```python
from build123d import *

# Parameters (mm, degrees)
F0_W     = 38.1
F0_H     = 25.4
F0_R     = 2.286
F1_DEPTH = 304.8
F2_R     = 12.7
F3_DEPTH = 25.401


with BuildPart() as f1:
    # F0 (on Front) → F1 (new body)
    with BuildSketch(Plane.XZ):
        with Locations((19.05, 12.7)):
            Rectangle(F0_W, F0_H)
        with Locations((9.906, 12.7)):
            Circle(F0_R, mode=Mode.SUBTRACT)
        with Locations((28.194, 12.7)):
            Circle(F0_R, mode=Mode.SUBTRACT)
    extrude(amount=F1_DEPTH)

    # F2 (on Top) → F3 (cut, through all)
    with BuildSketch(Plane.XY):
        with Locations((17.78, -241.3)):
            Circle(F2_R)
        with Locations((17.78, -63.5)):
            Circle(F2_R)
    extrude(amount=F3_DEPTH, mode=Mode.SUBTRACT)


solid = f1.part
```
Model file for the job. Use its own axes, mm. Coordinates: 2 decimals unless noted, no trailing zeros. Loops run counter-clockwise (first coordinate to the right, second up) from the corner with the lowest first, then second, coordinate; pieces in that order, holes last. Notation, with made-up numbers: (24, 4) - (77, 4) arc R31 cw to (77, 31) - close; hole circle Ø3 at (-14.75, 83). An arc over 180 degrees is marked (long way). Write item = value, one per line. Start each with the question number.
Item 1: Saw through at A-A, the plane x = 17.78. List the corners of the cut face in (y, z), then the cut area to 3 significant figures.
Item 2: Drop a flat-ended pin along its axis: pin 1 Ø5.5 at (x, z) = (28.194, 12.7) entering from -Y. Give the stop position or say it passes through.
Item 3: Saw through at B-B, the plane y = -150. List the corners of the cut face in (x, z), then the cut area to 3 significant figures.
Item 4: Wall check: probe 1 along Y at (x, z) = (18, 19.5); probe 2 along X at (y, z) = (-257, 13); probe 3 along X at (y, z) = (-216.5, 12.25). Give the ranges that are in metal, low to high. Write a range as [from, to].
Item 5: Saw through at C-C, the plane z = 22.75. List the corners of the cut face in (x, y), then the cut area to 3 significant figures.
Item 6: Pull direction X, two halves, no side cores. Call faces 1 (the face through (0, -150, 13)), 2 (the face through (5.092, -240.742, 12.522)), 3 (the face through (19, -150, 0)): +X half, -X half, draft (parallel to the pull), parting line (faces both ways), or undercut.
Answers:
q1.outline = (-304.8, 0) - (-254, 0) - (-254, 25.4) - (-304.8, 25.4) - close; (-228.6, 0) - (-76.2, 0) - (-76.2, 25.4) - (-228.6, 25.4) - close; (-50.8, 0) - (0, 0) - (0, 25.4) - (-50.8, 25.4) - close
q1.area = 6,450 mm2
q2.pin_1 = -304.8
q3.outline = (0, 0) - (38.1, 0) - (38.1, 25.4) - (0, 25.4) - close; hole circle Ø4.57 at (9.91, 12.7); hole circle Ø4.57 at (28.19, 12.7)
q3.area = 935 mm2
q4.probe_1 = [-304.8, -254], [-228.6, -76.2], [-50.8, 0]
q4.probe_2 = [0, 7.64], [12.17, 25.93], [30.46, 38.1]
q4.probe_3 = [0, 7.66], [12.15, 25.95], [30.44, 38.1]
q5.outline = (0, -304.8) - (38.1, -304.8) - (38.1, 0) - (0, 0) - close; hole circle Ø25.4 at (17.78, -241.3); hole circle Ø25.4 at (17.78, -63.5)
q5.area = 10,600 mm2
q6.face_1 = -X half
q6.face_2 = undercut
q6.face_3 = draft
